```python
from build123d import *

# Parameters (mm, degrees)
SKETCH_R        = 1.75
PAD_DEPTH       = 24.5
SKETCH001_W     = 15
SKETCH001_H     = 12
POCKET_DEPTH    = 14.5
SKETCH002_W     = 20
SKETCH002_H     = 20
POCKET001_DEPTH = 19.5
SKETCH003_R     = 2.6
POCKET002_DEPTH = 24.501
POCKET003_DEPTH = 20.001
FILLET_R        = 0.5


with BuildPart() as part:
    # Sketch → Pad (new body)
    with BuildSketch(Plane.XY):
        with BuildLine():
            Line((-2.130082, 4.523577), (9.5, 10))
            Line((9.5, 10), (34, 10))
            Line((34, 10), (34, 2.6))
            Line((24.5, 2.6), (34, 2.6))
            ThreePointArc((24.5, 2.6), (21.9, 0), (24.5, -2.6))
            Line((24.5, -2.6), (34, -2.6))
            Line((34, -2.6), (34, -10))
            Line((34, -10), (9.5, -10))
            Line((9.5, -10), (-2.130082, -4.523577))
            ThreePointArc((-2.130082, 4.523577), (-5, 0), (-2.130082, -4.523577))
        make_face()
        Circle(SKETCH_R, mode=Mode.SUBTRACT)
    extrude(amount=PAD_DEPTH)

    # Sketch001 (on Face12 of Pad) → Pocket (cut)
    with BuildSketch(Plane(origin=(0, 0, 0), x_dir=(1, 0, 0), z_dir=(0, 0, -1))):
        with Locations((2, 0)):
            Rectangle(SKETCH001_W, SKETCH001_H)
    extrude(amount=-POCKET_DEPTH, mode=Mode.SUBTRACT)

    # Sketch002 (on Face4 of Pocket) → Pocket001 (cut)
    with BuildSketch(Plane(origin=(0, 0, 0), x_dir=(1, 0, 0), z_dir=(0, 0, -1))):
        with Locations((24.5, 0)):
            Rectangle(SKETCH002_W, SKETCH002_H)
    extrude(amount=-POCKET001_DEPTH, mode=Mode.SUBTRACT)

    # Sketch003 (on Face9 of Pocket001) → Pocket002 (cut, through all)
    with BuildSketch(Plane(origin=(9.5, 0, 0), x_dir=(0, -1, 0), z_dir=(-1, 0, 0))):
        with Locations((0, 9.5)):
            Circle(SKETCH003_R)
    extrude(amount=-POCKET002_DEPTH, mode=Mode.SUBTRACT)

    # Sketch004 (on Face5 of Pocket002) → Pocket003 (cut, through all)
    with BuildSketch(Plane(origin=(0, 10, 0), x_dir=(-1, 0, 0), z_dir=(0, 1, 0))):
        Polygon((-8.9, 0), (-4, 14.49), (0, 14.49), (0, 0), align=None)
    extrude(amount=-POCKET003_DEPTH, mode=Mode.SUBTRACT)

    # Fillet
    fillet_edges = [part.edges().sort_by_distance(p)[0] for p in [
        (6.45, -8.563803, 7.245),
        (6.45, -6, 7.245),
        (6.45, 6, 7.245),
        (6.45, 8.563803, 7.245),
        (14.5, -10, 9.75),
        (14.5, 10, 9.75),
        (34, -2.6, 22),
        (34, 2.6, 22),
        (9.5, -10, 12.25),
        (9.5, 10, 12.25),
        (34, -10, 22),
        (34, 10, 22),
    ]]
    fillet(fillet_edges, radius=FILLET_R)


solid = part.part
```
The model under review builds one solid part; all positions refer to its coordinate system, in mm. A direction names the side the tool comes from. Round coordinates to 2 decimals unless told otherwise and drop trailing zeros. Loops run counter-clockwise (first coordinate to the right, second up) from the corner with the lowest first, then second, coordinate; pieces in that order, holes last. Notation, with made-up numbers: (76.25, -14) -> (85.25, -14) arc R6 cw to (85.25, -6) -> close; hole circle Ø3 at (19, 33). An arc over 180 degrees is marked (long way). Answer as a JSON object with one key per item and string values. Group by question number.
1) We need section D-D on x = 0. Write out the cut boundary in (y, z), then the cut area to 3 significant figures.
2) For faces 1 (the face through (14.5, 2, 12)), 2 (the face through (8, -6, 9)), 3 (the face through (29, -2.6, 22)), list the 3-axis set-ups (+Z, -Z, +X, -X, +Y, -Y) from which the entire face can be reached by the end or side of a thin tool; tool diameter is ignored.
3) We need section C-C on x = 13.5. Write out the cut boundary in (y, z).
4) We need section A-A on x = 26.5. Write out the cut boundary in (y, z), then the cut area to 3 significant figures.
5) We need section B-B on y = 0. Write out the cut boundary in (x, z), then the cut area to 4 significant figures.
6) Mouldability with a two-part tool opening along Y and no side actions: class faces 4 (the face through (21.6, -0.1, 19.5)), 5 (the face through (1.617, -0.67, 19.43)), 6 (the face through (9.5, 0, 6)), 7 (the face through (13, 10, 18)) as released by +Y, released by -Y, zero draft, split by the parting line, or undercut.
7) For pin 1 Ø2 at (y, z) = (1, 12.5) entering from -X; pin 2 Ø0.8 at (x, y) = (2, -7) entering from -Z; pin 3 Ø7 at (x, z) = (6, 7) entering from +Y; pin 4 Ø1.2 at (x, y) = (2, 6.5) entering from -Z, all flat-tipped, find the tip position at first contact; note any pin that passes through.
8) For line 1 (X direction, y = 0, z = 19); line 2 (X direction, y = 0, z = 20.25); line 3 (X direction, y = -5, z = 7), list the stretches that pass through material, from the lowest coordinate up. Write a range as [from, to].
Result set:
{
 "1": {"outline": "(-5.53, 14.5) -> (-1.75, 14.5) -> (-1.75, 24.5) -> (-5.53, 24.5) -> close; (1.75, 14.5) -> (5.53, 14.5) -> (5.53, 24.5) -> (1.75, 24.5) -> close", "area": "75.5 mm²"},
 "2": {"face 1": "-Z, +X, +Y, -Y", "face 2": "-Z, -X", "face 3": "+Z, -Z, +X"},
 "3": {"outline": "(-10, 0) -> (10, 0) -> (10, 24.5) -> (-10, 24.5) -> close; hole circle Ø5.2 at (0, 9.5)"},
 "4": {"outline": "(-10, 19.5) -> (-2.6, 19.5) -> (-2.6, 24.5) -> (-10, 24.5) -> close; (2.6, 19.5) -> (10, 19.5) -> (10, 24.5) -> (2.6, 24.5) -> close", "area": "74.0 mm²"},
 "5": {"outline": "(-5, 14.5) -> (-1.75, 14.5) -> (-1.75, 24.5) -> (-5, 24.5) -> close; (1.75, 14.5) -> (9.5, 14.5) -> (9.5, 12.1) -> (14.5, 12.1) -> (14.5, 19.5) -> (21.9, 19.5) -> (21.9, 24.5) -> (1.75, 24.5) -> close; (9.5, 0) -> (14.5, 0) -> (14.5, 6.9) -> (9.5, 6.9) -> close", "area": "243.5 mm²"},
 "6": {"face 4": "zero draft", "face 5": "undercut", "face 6": "undercut", "face 7": "released by +Y"},
 "7": {"pin 1": "x = 9.5", "pin 2": "through", "pin 3": "y = 9.99", "pin 4": "z = 14.49"},
 "8": {"line 1": "[-5, -1.75], [1.75, 14.5]", "line 2": "[-5, -1.75], [1.75, 21.9]", "line 3": "[9.5, 14.5]"}
}
